Input: part model. Units: mm. Frame: model coordinates. A direction names the side the tool comes from. Round coordinates to 2 decimals unless told otherwise and drop trailing zeros. Loops run counter-clockwise (first coordinate to the right, second up) from the corner with the lowest first, then second, coordinate; pieces in that order, holes last. Notation, with made-up numbers: (-19, 42.25) - (20, 42.25) arc R20 cw to (20, 74.25) - close; hole circle Ø10 at (-3.75, -2.5). An arc over 180 degrees is marked (long way). Write each question's results on one line, items separated by ' | '.
from build123d import *

# Parameters (mm, degrees)
SKETCH3_W           = 34.39206684
SKETCH3_H           = 13.864626052
SKETCH3_R           = 1.948262706
BOSS_EXTRUDE1_DEPTH = 4
CUT_EXTRUDE2_DEPTH  = 2


with BuildPart() as part:
    # Sketch3 → Boss-Extrude1 (new body)
    with BuildSketch(Plane(origin=(0, 0, 0), x_dir=(-1, 0, 0), z_dir=(0, 0, 1))):
        with Locations((-14.628449162, 10.554141489)):
            Rectangle(SKETCH3_W, SKETCH3_H)
        with Locations(Location((-26.628449162, 10.547774914, 0), (0, 0, 180))):
            Circle(SKETCH3_R, mode=Mode.SUBTRACT)
        with Locations(Location((-2.628449162, 10.547774914, 0), (0, 0, 180))):
            Circle(SKETCH3_R, mode=Mode.SUBTRACT)
    extrude(amount=BOSS_EXTRUDE1_DEPTH)

    # Sketch4 → Cut-Extrude2 (cut)
    with BuildSketch(Plane.XY.offset(4)):
        Polygon((3.987302292, -3.609095314), (-2.567584258, -3.609095314), (-2.567584258, -17.486454515), (3.987302292, -17.486454515), (0.680186456, -10.547774914), align=None)
        Polygon((25.128096542, -3.609095314), (31.824482582, -3.609095314), (31.824482582, -17.486454515), (25.128096542, -17.486454515), (28.476289562, -10.547774914), align=None)
    extrude(amount=-CUT_EXTRUDE2_DEPTH, mode=Mode.SUBTRACT)


solid = part.part
1. Line query: line 1 (X direction, y = -10.5, z = 0.95); line 2 (X direction, y = -10.5, z = 2.85); line 3 (X direction, y = -12.25, z = 1.8). Output: solid intervals per line, ascending. Write a range as [from, to].
Answer:
line 1: [-2.57, 0.68], [4.58, 24.68], [28.58, 31.82] | line 2: [4.58, 24.68] | line 3: [-2.57, 1.68], [3.58, 25.68], [27.58, 31.82]
2. Contact query for flat-ended pins moving along their axis: pin 1 (2 mm diameter, centred on x = 30, y = -7, fed in from +Z); pin 2 (2 mm diameter, centred on y = -8, z = 3.5, fed in from +X); pin 3 (3 mm diameter, centred on x = 26.63, y = -10.55, fed in from +Z). Output: stop coordinate, or through.
Answer:
pin 1: z = 2 | pin 2: x = 27.69 | pin 3: through
3. Section query C-C, the plane y = -15.5. Output: boundary loops of the cut face in (x, z).
Answer:
outline: (-2.57, 0) - (31.82, 0) - (31.82, 2) - (26.09, 2) - (26.09, 4) - (3.04, 4) - (3.04, 2) - (-2.57, 2) - close
4. Section query A-A, the plane y = -11. Output: boundary loops of the cut face in (x, z).
Answer:
outline: (-2.57, 0) - (0.73, 0) - (0.73, 2) - (-2.57, 2) - close; (4.52, 0) - (24.73, 0) - (24.73, 4) - (4.52, 4) - close; (28.52, 0) - (31.82, 0) - (31.82, 2) - (28.52, 2) - close
5. Mould query, pull axis Y, two halves, no side actions, for faces 1 (the cylindrical face through (24.682, -10.462, 1.972)), 2 (the cylindrical face through (4.43, -11.29, 1.97)), 3 (the flat face through (26.39, -14.87, 3.01)), 4 (the flat face through (29, -10, 2)). Classes: pulls with the +Y half, pulls with the -Y half, needs draft (parallel to the pull), parting line crosses it, or undercut.
Answer:
face 1: undercut | face 2: undercut | face 3: pulls with the -Y half | face 4: needs draft
6. Section query D-D, the plane y = -5.25. Output: boundary loops of the cut face in (x, z).
Answer:
outline: (-2.57, 0) - (31.82, 0) - (31.82, 2) - (25.92, 2) - (25.92, 4) - (3.21, 4) - (3.21, 2) - (-2.57, 2) - close
7. Section query B-B, the plane z = 1.65. Output: boundary loops of the cut face in (x, y), plus the area to 3 significant figures.
Answer:
outline: (-2.57, -17.49) - (31.82, -17.49) - (31.82, -3.62) - (-2.57, -3.62) - close; hole circle Ø3.9 at (2.63, -10.55); hole circle Ø3.9 at (26.63, -10.55) | area: 453 mm^2
8. Set-up query: faces 5 (the flat face through (26.429, -6.304, 3.014)), 6 (the flat face through (15, -17.486, 2)), 7 (the flat face through (2.67, -6.37, 3.01)), 8 (the flat face through (2.71, -14.81, 3.01)). Return all of +Z, -Z, +X, -X, +Y, -Y with unobstructed straight access to the full face (end or side cutting, diameter ignored); none if empty.
Answer:
face 5: +Z, +X, +Y | face 6: +Z, -Z, +X, -X, -Y | face 7: +Z, -X, +Y | face 8: +Z, -X, -Y
